```python
from build123d import *

# Parameters (mm, degrees)
F1_DEPTH = 88.9
F3_D     = 31.75
F5_D     = 3.175


with BuildPart() as f1:
    # F0 (on Front) → F1 (new body)
    with BuildSketch(Plane.XZ):
        Polygon((0, 76.2), (0, 0), (25.4, 0), (25.4, 3.175), (3.175, 3.175), (3.175, 76.2), align=None)
    extrude(amount=F1_DEPTH)

    # F3 (through all)
    with Locations(Plane(origin=(0, 0, 0), x_dir=(0, -1, 0), z_dir=(-1, 0, 0))):
        with Locations((44.45, 38.1)):
            Hole(F3_D / 2)

    # F5 (through all)
    with Locations(Plane(origin=(0, 0, 0), x_dir=(1, 0, 0), z_dir=(0, 0, -1))):
        with Locations((12.7, 82.55), (12.7, 57.15), (12.7, 31.75), (12.7, 6.35)):
            Hole(F5_D / 2)


solid = f1.part
```
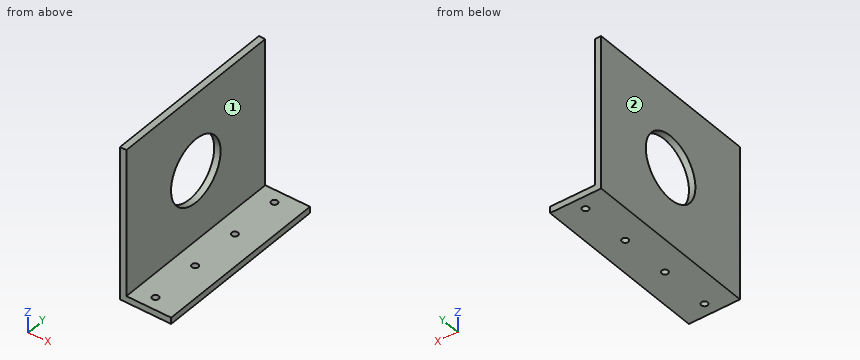
Can you work these out from the model? Positions are in its coordinate system, mm. Face numbers are marked on the shaded views. A direction names the side the tool comes from. Round coordinates to 2 decimals unless told otherwise and drop trailing zeros. Loops run counter-clockwise (first coordinate to the right, second up) from the corner with the lowest first, then second, coordinate; pieces in that order, holes last. Notation, with made-up numbers: M 46,11.5 L 78,11.5 A9 cw 78,17.5 Z; hole C 5.5,78.5 d11. An arc over 180 degrees is marked long. Write item = value, one per line. Start each with the question number.
(1) Suppose I cut it at B-B on x = 12.7. Write out the boundary of the cut face in (y, z) (1 decimal).
(2) Suppose I cut it at A-A on y = -82.55. Write out the boundary of the cut face in (x, z) (1 decimal).
(3) Which directions (+Z, -Z, +X, -X, +Y, -Y) give clear straight access to the entire face, cutting with the end or side of a thin tool? Please do the marked faces 1 and 2.
(4) I need wall thicknesses on line 1 along Y through (x, z) = (12.7, 1.15); line 2 along X through (y, z) = (-6.35, 1.65); line 3 along Z through (x, y) = (5.75, -26.5) (3 decimals). Which ranges of each line are inside material? Lowest first, please.
(5) Suppose I cut it at C-C on z = 38.1. Write out the boundary of the cut face in (x, y) (3 decimals), plus the area to 3 significant figures.
(6) Suppose I cut it at D-D on y = -24.5. Write out the boundary of the cut face in (x, z) (3 decimals).
(7) I'm going to push flat-ended pins straight in: P1, Ø4, axis at y = -63.5, z = 58, coming from the +X side (3 decimals); P2, Ø4, axis at x = 10.5, y = -49.5, coming from the +Z side (3 decimals). Where does each tip first touch, or does it pass through?
Answer block:
q1.outline = M -88.9,0 L -84.1,0 L -84.1,3.2 L -88.9,3.2 Z; M -81,0 L -58.7,0 L -58.7,3.2 L -81,3.2 Z; M -55.6,0 L -33.3,0 L -33.3,3.2 L -55.6,3.2 Z; M -30.2,0 L -7.9,0 L -7.9,3.2 L -30.2,3.2 Z; M -4.8,0 L 0,0 L 0,3.2 L -4.8,3.2 Z
q2.outline = M 0,0 L 11.1,0 L 11.1,3.2 L 3.2,3.2 L 3.2,76.2 L 0,76.2 Z; M 14.3,0 L 25.4,0 L 25.4,3.2 L 14.3,3.2 Z
q3.face_1 = +Z, +X, +Y, -Y
q3.face_2 = +Z, -Z, -X, +Y, -Y
q4.line_1 = -88.9 to -84.14, -80.96 to -58.74, -55.56 to -33.34, -30.16 to -7.94, -4.76 to 0
q4.line_2 = 0 to 11.11, 14.29 to 25.4
q4.line_3 = 0 to 3.175
q5.outline = M 0,-88.9 L 3.175,-88.9 L 3.175,-60.325 L 0,-60.325 Z; M 0,-28.575 L 3.175,-28.575 L 3.175,0 L 0,0 Z
q5.area = 181 mm²
q6.outline = M 0,0 L 25.4,0 L 25.4,3.175 L 3.175,3.175 L 3.175,76.2 L 0,76.2 Z
q7.P1 = 3.175
q7.P2 = 3.175
